Build history of the part. All positions in model axes, mm. A direction names the side the tool comes from. Coordinates: 2 decimals unless noted, no trailing zeros. Loops run counter-clockwise (first coordinate to the right, second up) from the corner with the lowest first, then second, coordinate; pieces in that order, holes last.
Item 1: Flat gauge pins, fed straight in: pin 1 (2 mm diameter, centred on x = -9, y = 5.5, fed in from +Z); pin 2 (8 mm diameter, centred on y = 6.5, z = 2, fed in from -X); pin 3 (8 mm diameter, centred on x = -4.5, z = 5.5, fed in from +Y). Where does each tip first touch, or does it go through?
Item 2: Drill centre lines: line 1 along X through (y, z) = (5.5, 1.5); line 2 along Z through (x, y) = (3.75, -6.75); line 3 along Y through (x, z) = (8, 1.2). Where is each one in solid material? Low to high.
Item 3: Cut at C-C (y = -8). List the corners of the cut face in (x, z).
Item 4: Cut at A-A (x = 0). List the corners of the cut face in (y, z).
Item 5: Mould opens along X. For faces 1 (the face through (-3, 3, 3)), 2 (the face through (2.02, -3.16, 10.49)), 3 (the face through (-0.238, 6.926, 1.479)) say: released by +X, released by -X, zero draft, split by the parting line, or undercut.
Item 6: 3-axis set-ups, long thin cutter, end or side, ignore diameter. For faces 4 (the face through (-0.878, -3.954, 12.726)), 5 (the face through (11.923, 3.755, 1.479)): which of +Z, -Z, +X, -X, +Y, -Y reach the whole face in a straight line?
from build123d import *

# Parameters (mm, degrees)
SKETCH1_R           = 12.5
SKETCH1_R_2         = 1.1
BOSS_EXTRUDE1_DEPTH = 3
SKETCH2_R           = 4.05
BOSS_EXTRUDE2_DEPTH = 12
SKETCH3_W           = 1
SKETCH3_H           = 0.6
FILLET1_SIZE        = 0.5


with BuildPart() as part:
    # Sketch1 → Boss-Extrude1 (new body)
    with BuildSketch(Plane.XY):
        Circle(SKETCH1_R)
        with Locations((0, 8)):
            Circle(SKETCH1_R_2, mode=Mode.SUBTRACT)
        with Locations((5.656854249, 5.656854249)):
            Circle(SKETCH1_R_2, mode=Mode.SUBTRACT)
        with Locations((8, 0)):
            Circle(SKETCH1_R_2, mode=Mode.SUBTRACT)
        with Locations((5.656854249, -5.656854249)):
            Circle(SKETCH1_R_2, mode=Mode.SUBTRACT)
        with Locations((0, -8)):
            Circle(SKETCH1_R_2, mode=Mode.SUBTRACT)
        with Locations((-5.656854249, -5.656854249)):
            Circle(SKETCH1_R_2, mode=Mode.SUBTRACT)
        with Locations((-8, 0)):
            Circle(SKETCH1_R_2, mode=Mode.SUBTRACT)
        with Locations((-5.656854249, 5.656854249)):
            Circle(SKETCH1_R_2, mode=Mode.SUBTRACT)
    extrude(amount=BOSS_EXTRUDE1_DEPTH)

    # Sketch2 → Boss-Extrude2 (add)
    with BuildSketch(Plane.XY.offset(3)):
        Circle(SKETCH2_R)
    extrude(amount=BOSS_EXTRUDE2_DEPTH)

    # Sketch3 → Cut-Revolve1 (revolve, cut)
    with BuildSketch(Plane(origin=(0, 0, 0), x_dir=(0, 0, -1), z_dir=(1, 0, 0)), mode=Mode.PRIVATE) as cut_revolve1_sk:
        with Locations((-10.5, 4.05)):
            Rectangle(SKETCH3_W, SKETCH3_H)
    revolve(cut_revolve1_sk.sketch.rotate(Axis((0, 0, 15), (0, 0, -1)), 90), axis=Axis((0, 0, 15), (0, 0, -1)), mode=Mode.SUBTRACT)

    # Fillet1
    fillet1_edges = [part.edges().sort_by_distance(p)[0] for p in [
        (-4.05, 0, 15),
    ]]
    chamfer(fillet1_edges, length=FILLET1_SIZE)


solid = part.part
Filled sheet:
1. pin 1: stops at z = 3
1. pin 2: stops at x = -12.25
1. pin 3: stops at y = 12.42
2. line 1: x = -11.22 to -6.75, -4.57 to 4.57, 6.75 to 11.22
2. line 2: z = 0 to 3
2. line 3: y = -9.6 to -1.1, 1.1 to 9.6
3. outline: (-9.6, 0) - (-1.1, 0) - (-1.1, 3) - (-9.6, 3) - close; (1.1, 0) - (9.6, 0) - (9.6, 3) - (1.1, 3) - close
4. outline: (-12.5, 0) - (-9.1, 0) - (-9.1, 3) - (-12.5, 3) - close; (-6.9, 0) - (6.9, 0) - (6.9, 3) - (4.05, 3) - (4.05, 10) - (3.75, 10) - (3.75, 11) - (4.05, 11) - (4.05, 14.5) - (3.55, 15) - (-3.55, 15) - (-4.05, 14.5) - (-4.05, 11) - (-3.75, 11) - (-3.75, 10) - (-4.05, 10) - (-4.05, 3) - (-6.9, 3) - close; (9.1, 0) - (12.5, 0) - (12.5, 3) - (9.1, 3) - close
5. face 1: zero draft
5. face 2: split by the parting line
5. face 3: undercut
6. face 4: +Z
6. face 5: +Z, -Z
